```python
from build123d import *

# Parameters (mm, degrees)
SKETCH1_W               = 88.9
SKETCH1_H               = 88.9
BASE_DRAIN_TRAY_DEPTH   = 10.16
SKETCH2_W               = 86.36
SKETCH2_H               = 86.36
DRAIN_TRAY_CUTOUT_DEPTH = 8.89
SKETCH3_W               = 71.12
SKETCH3_H               = 71.12
BODY_DEPTH              = 50.8
SKETCH4_W               = 68.58
SKETCH4_H               = 68.58
BODY_CUTOUT_DEPTH       = 50.8
FILLET1_R               = 1.27
JOINING_SLOT_DEPTH      = 8.89
JOINING_CUTOUT_DEPTH    = 8.89
JOINING_SLOT_2_DEPTH    = 8.89
JOINING_CUTOUT_2_DEPTH  = 8.89
BOSS_EXTRUDE3_DEPTH     = 8.89
SKETCH14_W              = 71.12
SKETCH14_H              = 71.12
CUT_EXTRUDE2_DEPTH      = 50.8


with BuildPart() as part:
    # Sketch1 → Base/Drain Tray (new body)
    with BuildSketch(Plane(origin=(0, 0, 0), x_dir=(1, 0, 0), z_dir=(0, 1, 0))):
        with Locations((44.45, 44.45)):
            Rectangle(SKETCH1_W, SKETCH1_H)
    extrude(amount=BASE_DRAIN_TRAY_DEPTH)

    # Sketch2 → Drain Tray Cutout (cut)
    with BuildSketch(Plane(origin=(0, 10.16, 0), x_dir=(1, 0, 0), z_dir=(0, 1, 0))):
        with Locations((44.45, 44.45)):
            Rectangle(SKETCH2_W, SKETCH2_H)
    extrude(amount=-DRAIN_TRAY_CUTOUT_DEPTH, mode=Mode.SUBTRACT)

    # Sketch3 → Body (add)
    with BuildSketch(Plane(origin=(0, 1.27, 0), x_dir=(1, 0, 0), z_dir=(0, 1, 0))):
        with Locations((44.45, 44.45)):
            Rectangle(SKETCH3_W, SKETCH3_H)
    extrude(amount=BODY_DEPTH)

    # Sketch4 → Body Cutout (cut)
    with BuildSketch(Plane(origin=(0, 52.07, 0), x_dir=(1, 0, 0), z_dir=(0, 1, 0))):
        with Locations((44.45, 44.45)):
            Rectangle(SKETCH4_W, SKETCH4_H)
    extrude(amount=-BODY_CUTOUT_DEPTH, mode=Mode.SUBTRACT)

    # Fillet1
    fillet1_edges = [part.edges().sort_by_distance(p)[0] for p in [
        (0, 5.08, -88.9),
        (88.9, 5.08, -88.9),
        (88.9, 5.08, 0),
        (0, 5.08, 0),
    ]]
    fillet(fillet1_edges, radius=FILLET1_R)

    # Sketch7 → Joining Slot (add)
    with BuildSketch(Plane(origin=(0, 1.27, 0), x_dir=(1, 0, 0), z_dir=(0, 1, 0))):
        Polygon((40.64, 85.09), (41.486666667, 87.63), (39.478620352, 87.63), (37.996953686, 83.185), (50.903046314, 83.185), (49.421379648, 87.63), (47.413333333, 87.63), (48.26, 85.09), align=None)
    extrude(amount=JOINING_SLOT_DEPTH)

    # Sketch8 → Joining Cutout (cut)
    with BuildSketch(Plane(origin=(0, 10.16, 0), x_dir=(1, 0, 0), z_dir=(0, 1, 0))):
        Polygon((40.64, 85.09), (41.486666667, 87.63), (41.91, 88.9), (46.99, 88.9), (47.413333333, 87.63), (48.26, 85.09), align=None)
    extrude(amount=-JOINING_CUTOUT_DEPTH, mode=Mode.SUBTRACT)

    # Sketch10 → Joining Slot 2 (add)
    with BuildSketch(Plane(origin=(0, 1.27, 0), x_dir=(1, 0, 0), z_dir=(0, 1, 0))):
        Polygon((87.63, 49.421379648), (87.63, 39.478620352), (83.185, 37.996953686), (83.185, 50.903046314), align=None)
    extrude(amount=JOINING_SLOT_2_DEPTH)

    # Sketch12 → Joining Cutout 2 (cut)
    with BuildSketch(Plane(origin=(0, 1.27, 0), x_dir=(1, 0, 0), z_dir=(0, 1, 0))):
        Polygon((88.9, 41.91), (88.9, 46.99), (85.09, 48.26), (85.09, 40.64), align=None)
    extrude(amount=JOINING_CUTOUT_2_DEPTH, mode=Mode.SUBTRACT)

    # Sketch13 → Boss-Extrude3 (add)
    with BuildSketch(Plane(origin=(0, 1.27, 0), x_dir=(1, 0, 0), z_dir=(0, 1, 0))):
        Polygon((42.037, 0), (46.863, 0), (48.006, -3.556), (44.45, -3.556), (40.894, -3.556), align=None)
        Polygon((0, 46.863), (0, 42.037), (-3.556, 40.894), (-3.556, 44.45), (-3.556, 48.006), align=None)
    extrude(amount=BOSS_EXTRUDE3_DEPTH)

    # Sketch14 → Cut-Extrude2 (cut)
    with BuildSketch(Plane(origin=(0, 52.07, 0), x_dir=(1, 0, 0), z_dir=(0, 1, 0))):
        with Locations((44.45, 44.45)):
            Rectangle(SKETCH14_W, SKETCH14_H)
    extrude(amount=-CUT_EXTRUDE2_DEPTH, mode=Mode.SUBTRACT)


solid = part.part
```
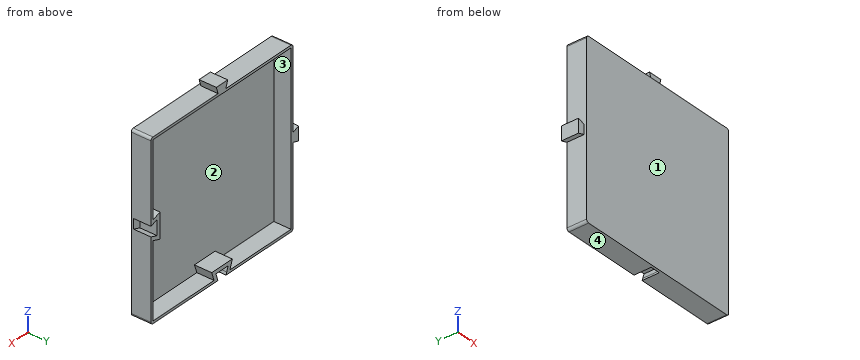
The model under review builds one solid part; all positions refer to its coordinate system, in mm. Face numbers are marked on the shaded views. Coordinates: 2 decimals unless noted, no trailing zeros. Write each loop counter-clockwise with the first axis right and the second up, starting at its lowest first coordinate (ties: lowest second). Pieces come first, ordered by that corner, then holes.
1) We need section A-A on x = 5.5. State the section outline as (y, z) points, then the cut area to 3 significant figures.
2) Clearance check with flat-ended pins moving along their axes: pin 1 Ø4 at (y, z) = (7.5, -42.5) entering from +X; pin 2 Ø1 at (y, z) = (7.5, -58.5) entering from -X; pin 3 Ø1.1 at (x, z) = (-1, -43) entering from -Y; pin 4 Ø1 at (x, z) = (79.5, -27.5) entering from +Y. State where each tip first meets the part, or that it passes through.
3) To check wall thickness, follow probe 1 along X at (y, z) = (2, -63.5); probe 2 along Z at (x, y) = (17.5, 3.5); probe 3 along X at (y, z) = (7.5, -43) (3 decimals). State the ranges of each line that lie inside material, in increasing order.
4) The part is to be moulded in two halves that separate along Z. For the marked faces 1, 2, 3 and 4, say which applies: pulls with the +Z half, pulls with the -Z half, needs draft (parallel to the pull), parting line crosses it, or undercut.
5) We need section B-B on z = -4.5. State the section outline as (x, y) points, then the cut area to 3 significant figures.
Answer list:
1. outline: (0, -88.9) - (10.16, -88.9) - (10.16, -87.63) - (1.27, -87.63) - (1.27, -1.27) - (10.16, -1.27) - (10.16, 0) - (0, 0) - close
1. area: 135 mm2
2. pin 1: stops at x = 88.9
2. pin 2: stops at x = 0
2. pin 3: stops at y = 1.27
2. pin 4: stops at y = 1.27
3. probe 1: x = 0 to 1.27, 87.63 to 88.9
3. probe 2: z = -88.9 to -87.63, -1.27 to 0
3. probe 3: x = -3.556 to 1.27, 83.185 to 85.09
4. face 1: needs draft
4. face 2: undercut
4. face 3: undercut
4. face 4: pulls with the -Z half
5. outline: (0, 0) - (88.9, 0) - (88.9, 10.16) - (87.63, 10.16) - (87.63, 1.27) - (1.27, 1.27) - (1.27, 10.16) - (0, 10.16) - close
5. area: 135 mm2
